```python
from build123d import *

# Parameters (mm, degrees)
BOSS_EXTRUDE1_DEPTH = 7
SKETCH1_4_R         = 4.75
BOSS_EXTRUDE2_DEPTH = 5


with BuildPart() as part:
    # Sketch1 → Boss-Extrude1 (new, symmetric)
    with BuildSketch(Plane(origin=(0, 0, 0), x_dir=(1, 0, 0), z_dir=(0, 1, 0))):
        with BuildLine():
            ThreePointArc((49.474147464, -4.374756762), (48.055615348, -2.58278673), (45.987853381, -1.609261996))
            Line((45.987853381, -1.609261996), (23.487853381, 3.173260641))
            ThreePointArc((23.487853381, 3.173260641), (18.171060665, 0.871975682), (18.596745327, -4.905825787))
            ThreePointArc((18.596745327, -4.905825787), (18.933207864, -7.564087513), (16.670970527, -9))
            Line((16.670970527, -9), (-50, -9))
            ThreePointArc((-50, -9), (-59, 0), (-50, 9))
            Line((-50, 9), (55, 9))
            ThreePointArc((55, 9), (57.828427125, 7.828427125), (59, 5))
            Line((59, 5), (59, -2.249513525))
            ThreePointArc((59, -2.249513525), (55.08874637, -7.129537228), (49.474147464, -4.374756762))
        make_face()
        with BuildLine():
            ThreePointArc((-50, 7), (-57, 0), (-50, -7))
            Line((-50, -7), (16.670970527, -7))
            ThreePointArc((16.670970527, -7), (17.123417995, -6.712817503), (17.056125487, -6.181165157))
            ThreePointArc((17.056125487, -6.181165157), (16.46016696, 1.9077569), (23.903676763, 5.129555843))
            Line((23.903676763, 5.129555843), (46.403676763, 0.347033205))
            ThreePointArc((46.403676763, 0.347033205), (49.298543517, -1.015901422), (51.284488478, -3.524659467))
            ThreePointArc((51.284488478, -3.524659467), (54.653247822, -5.177527747), (57, -2.249513525))
            Line((57, -2.249513525), (57, 5))
            ThreePointArc((57, 5), (56.414213562, 6.414213562), (55, 7))
            Line((55, 7), (-50, 7))
        make_face(mode=Mode.SUBTRACT)
    extrude(amount=BOSS_EXTRUDE1_DEPTH, both=True)

    # Sketch1_4 → Boss-Extrude2 (add, symmetric)
    with BuildSketch(Plane(origin=(0, 0, 0), x_dir=(1, 0, 0), z_dir=(0, 1, 0))):
        with BuildLine():
            Line((-50, 7), (55, 7))
            ThreePointArc((55, 7), (56.414213562, 6.414213562), (57, 5))
            Line((57, 5), (57, -2.249513525))
            ThreePointArc((57, -2.249513525), (54.653247822, -5.177527747), (51.284488478, -3.524659467))
            ThreePointArc((51.284488478, -3.524659467), (49.298543517, -1.015901422), (46.403676763, 0.347033205))
            Line((46.403676763, 0.347033205), (23.903676763, 5.129555843))
            ThreePointArc((23.903676763, 5.129555843), (16.46016696, 1.9077569), (17.056125487, -6.181165157))
            ThreePointArc((17.056125487, -6.181165157), (17.123417995, -6.712817503), (16.670970527, -7))
            Line((16.670970527, -7), (-50, -7))
            ThreePointArc((-50, -7), (-57, 0), (-50, 7))
        make_face()
        with Locations(Location((-50, 0, 0), (0, 0, 270))):
            Circle(SKETCH1_4_R, mode=Mode.SUBTRACT)
    extrude(amount=BOSS_EXTRUDE2_DEPTH, both=True)


solid = part.part
```
Verification items for the finished model (mm, model axes). A direction names the side the tool comes from. Give positions to 0.01 mm unless a question says otherwise; leave off trailing zeros. Loops run counter-clockwise (first coordinate to the right, second up) from the corner with the lowest first, then second, coordinate; pieces in that order, holes last. Notation, with made-up numbers: M 0.25,-34 L 19.25,-34 A28 ccw 19.25,-13 Z; hole C 3.25,13 d1. An arc over 180 degrees is marked long. One line per question, with ' | ' between items.
Item 1: Thickness scan on line 1 (Y direction, x = 12.5, z = -3); line 2 (X direction, y = -3.5, z = 6.25); line 3 (X direction, y = -1, z = 3). Record the ranges inside material, lowest first. Write a range as [from, to].
Completed:
line 1: y = [-5, 5] | line 2: x = [-56.48, 19.16], [51, 57] | line 3: x = [-58.49, -53.68], [-46.32, 17.62], [48.52, 58.94]
Item 2: Section check B-B, the plane y = 2. Record the cut outline in (x, z), plus the area to 3 significant figures.
Completed:
outline: M -50,-9 L 55,-9 A4 ccw 59,-5 L 59,2.25 A5 ccw 49.47,4.37 A5 cw 45.99,1.61 L 23.49,-3.17 A5 cw 18.6,4.91 A2.5 ccw 16.67,9 L -50,9 A9 ccw Z; hole C -50,0 d9.5 | area: 1,680 mm^2
Item 3: Section check C-C, the plane x = 43.5. Record the cut outline in (y, z).
Completed:
outline: M -7,-9 L 7,-9 L 7,-7 L 5,-7 L 5,-0.96 L 7,-0.96 L 7,1.08 L -7,1.08 L -7,-0.96 L -5,-0.96 L -5,-7 L -7,-7 Z
Item 4: Draft check along X on faces 5 (the face through (-57, 6, 0)), 6 (the face through (56.43, 6.01, -6.4)), 7 (the face through (57.797, 0.098, -7.859)), 8 (the face through (4.6, 7, -7.4)). Enter one of: +X half, -X half, draft (parallel to the pull), parting line (faces both ways), or undercut.
Completed:
face 5: undercut | face 6: undercut | face 7: +X half | face 8: draft
Item 5: Tool access check on faces 1 (the face through (18.95, 0.1, 7.53)), 2 (the face through (-16, 0, 9)), 3 (the face through (54.6, 6.01, 5.19)), 4 (the face through (3, -6, -7)). Record the directions out of +Z, -Z, +X, -X, +Y, -Y that give a thin tool (end or side, any length) a straight path to the whole face; none if there is none.
Completed:
face 1: +Y, -Y | face 2: +Z, +X, -X, +Y, -Y | face 3: +Y | face 4: -Y
Item 6: Depth check by flat-ended pin: P1, Ø2, axis at y = 5.5, z = -2.5, coming from the -X side; P2, Ø1.5, axis at y = -5, z = 2.5, coming from the -X side. Enter the tip coordinate at first touch or a pass-through.
Completed:
P1: stops at x = -58.87 | P2: stops at x = -58.83
Item 7: Section check A-A, the plane x = 8.5. Record the cut outline in (y, z).
Completed:
outline: M -7,-9 L 7,-9 L 7,-7 L 5,-7 L 5,7 L 7,7 L 7,9 L -7,9 L -7,7 L -5,7 L -5,-7 L -7,-7 Z
